Read the model definition and answer for the solid it produces. Units are mm, in the model's axes. Coordinates: 2 decimals unless noted, no trailing zeros. Write each loop counter-clockwise with the first axis right and the second up, starting at its lowest first coordinate (ties: lowest second). Pieces come first, ordered by that corner, then holes.
Item 1: Section C-C (y = -108) is taken. Give the vertices of the cut face in (x, z), then the cut area to 3 significant figures.
Item 2: Determine the mould class of faces 1 (the face through (-21.085, -1.306, 0.986)), 2 (the face through (42, -74, 2)) for opening direction X: released by +X, released by -X, zero draft, split by the parting line, or undercut.
Item 3: Section B-B (x = -38) is taken. Give the vertices of the cut face in (y, z).
Item 4: Section A-A (x = -26) is taken. Give the vertices of the cut face in (y, z).
Item 5: This flat-tipped pin is pushed along its axis until it touches: P1, Ø1, axis at y = -127.5, z = 1, coming from the -X side. Where does it stop, or does it pass through?
Item 6: Straight lines are drawn through the part: probe 1 along Y at (x, z) = (29.5, 1.65); probe 2 along Y at (x, z) = (-38.5, 1.45); probe 3 along X at (y, z) = (-128, 1.4). For each, find the intervals that lie inside material, in ascending order.
Item 7: Section D-D (z = 1.3) is taken. State how many separate pieces and enclosed holes the cut face has, then the cut area to 3 significant figures.
from build123d import *

# Parameters (mm, degrees)
SKETCH_1_R      = 1.5
SKETCH_1_R_2    = 3.121318996
SKETCH_1_W      = 5.05
SKETCH_1_H      = 2.05
SKETCH_1_W_2    = 2.05
SKETCH_1_H_2    = 5.05
EXTRUDE_1_DEPTH = 2


with BuildPart() as part:
    # 草图1 → 凸台-拉伸1 (new body)
    with BuildSketch(Plane.XY):
        Polygon((-56.111334712, -13.372248853), (31.071025228, -13.372248853), (31.071025228, -137.372248853), (-56.111334712, -137.372248853), (-56.111334712, -152.372248853), (62.919821756, -152.372248853), (62.919821756, 1.627751147), (-56.111334712, 1.627751147), align=None)
        with Locations((-19.586334712, -1.372248853)):
            Circle(SKETCH_1_R, mode=Mode.SUBTRACT)
        with Locations((20.413665288, -1.372248853)):
            Circle(SKETCH_1_R, mode=Mode.SUBTRACT)
        with Locations((-19.586334712, -149.372248853)):
            Circle(SKETCH_1_R, mode=Mode.SUBTRACT)
        with Locations((20.413665288, -149.372248853)):
            Circle(SKETCH_1_R, mode=Mode.SUBTRACT)
        with Locations((59.919821756, -97.372248853)):
            Circle(SKETCH_1_R, mode=Mode.SUBTRACT)
        with Locations((59.919821756, -57.372248853)):
            Circle(SKETCH_1_R, mode=Mode.SUBTRACT)
        with Locations((41.938665288, -93.678088908)):
            Circle(SKETCH_1_R_2, mode=Mode.SUBTRACT)
        with Locations((39.413665288, -1.372248853)):
            Rectangle(SKETCH_1_W, SKETCH_1_H, mode=Mode.SUBTRACT)
        with Locations((49.413665288, -1.372248853)):
            Rectangle(SKETCH_1_W, SKETCH_1_H, mode=Mode.SUBTRACT)
        with Locations((-48.586334712, -1.372248853)):
            Rectangle(SKETCH_1_W, SKETCH_1_H, mode=Mode.SUBTRACT)
        with Locations((-38.586334712, -1.372248853)):
            Rectangle(SKETCH_1_W, SKETCH_1_H, mode=Mode.SUBTRACT)
        with Locations((39.413665288, -149.372248853)):
            Rectangle(SKETCH_1_W, SKETCH_1_H, mode=Mode.SUBTRACT)
        with Locations((49.413665288, -149.372248853)):
            Rectangle(SKETCH_1_W, SKETCH_1_H, mode=Mode.SUBTRACT)
        with Locations((-48.586334712, -149.372248853)):
            Rectangle(SKETCH_1_W, SKETCH_1_H, mode=Mode.SUBTRACT)
        with Locations((-38.586334712, -149.372248853)):
            Rectangle(SKETCH_1_W, SKETCH_1_H, mode=Mode.SUBTRACT)
        with Locations((59.919821756, -38.372248853)):
            Rectangle(SKETCH_1_W_2, SKETCH_1_H_2, mode=Mode.SUBTRACT)
        with Locations((59.919821756, -28.372248853)):
            Rectangle(SKETCH_1_W_2, SKETCH_1_H_2, mode=Mode.SUBTRACT)
        with Locations((59.919821756, -126.372248853)):
            Rectangle(SKETCH_1_W_2, SKETCH_1_H_2, mode=Mode.SUBTRACT)
        with Locations((59.919821756, -116.372248853)):
            Rectangle(SKETCH_1_W_2, SKETCH_1_H_2, mode=Mode.SUBTRACT)
    extrude(amount=EXTRUDE_1_DEPTH)


solid = part.part
Established:
1. outline: (31.07, 0) - (62.92, 0) - (62.92, 2) - (31.07, 2) - close
1. area: 63.7 mm2
2. face 1: undercut
2. face 2: zero draft
3. outline: (-152.37, 0) - (-150.4, 0) - (-150.4, 2) - (-152.37, 2) - close; (-148.35, 0) - (-137.37, 0) - (-137.37, 2) - (-148.35, 2) - close; (-13.37, 0) - (-2.4, 0) - (-2.4, 2) - (-13.37, 2) - close; (-0.35, 0) - (1.63, 0) - (1.63, 2) - (-0.35, 2) - close
4. outline: (-152.37, 0) - (-137.37, 0) - (-137.37, 2) - (-152.37, 2) - close; (-13.37, 0) - (1.63, 0) - (1.63, 2) - (-13.37, 2) - close
5. P1: stops at x = 31.07
6. probe 1: y = -152.37 to -137.37, -13.37 to 1.63
6. probe 2: y = -152.37 to -150.4, -148.35 to -137.37, -13.37 to -2.4, -0.35 to 1.63
6. probe 3: x = 31.07 to 58.89, 60.94 to 62.92
7. separate pieces: 1
7. enclosed holes: 19
7. area: 7,320 mm2
